Geometry: final body of the model. Coordinates: model frame, mm. A direction names the side the tool comes from. Round coordinates to 2 decimals unless told otherwise and drop trailing zeros. Order: outer loops, then holes, each group sorted by start corner. A loop starts at its lowest first (then second) coordinate and runs counter-clockwise, first axis right, second up. Notation, with made-up numbers: M -37.5,-28.5 L -24.5,-28.5 A21 ccw -24.5,-11.5 Z; hole C 85.25,-30 d2. An arc over 180 degrees is marked long. Put each result on its own line as item: value. Start each with the question number.
1) Section C-C, the plane y = 13. Return loops of the section in (x, z).
2) Section B-B, the plane z = -8.75. Return loops of the section in (x, y).
3) First-contact query: P1, Ø6, axis at y = 26, z = -4, coming from the -X side; P2, Ø1.2, axis at x = 1.5, y = 32.5, coming from the -Z side; P3, Ø4, axis at y = 7.5, z = -12.2, coming from the -X side. Flat tips, straight axial feed; report the tip coordinate or a pass-through.
4) Material intervals for probe 1 along Y at (x, z) = (1.2, -7.5); probe 2 along Z at (x, y) = (-1.1, 20); probe 3 along Y at (x, z) = (1.4, -13), sorted ascending. Write a range as [from, to].
5) Section D-D, the plane x = -0.45. Return loops of the section in (y, z), then the cut area to 3 significant figures.
6) Access query for faces 4 (the flat face through (1.232, 34.936, -13.58)), 5 (the flat face through (1, 7, -9.4)), 6 (the cylindrical face through (-3.01, 4.96, -12.76)). Directions: +Z, -Z, +X, -X, +Y, -Y. A direction counts if a zero-diameter tool reaches every point of the face in a straight line with its end or side. Return the directions, or none.
7) Draft query along Z for faces 1 (the flat face through (1.232, 34.914, -10.78)), 2 (the flat face through (-2.5, 20.3, -5.7)), 3 (the flat face through (1, 32, -9.4)). Return one class per face: pulls with the +Z half, pulls with the -Z half, needs draft (parallel to the pull), parting line crosses it, or undercut.
8) Section A-A, the plane x = 1.2. Return loops of the section in (y, z), then the cut area to 3 significant figures.
from build123d import *
from build123d.topology import SkipClean

# Parameters (mm, degrees)
BOSS_EXTRUDE1_DEPTH = 2.5
BOSS_EXTRUDE2_START = -2.5
SKETCH1_3_W         = 15
SKETCH1_3_H         = 40
SKETCH1_3_R         = 1.6
BOSS_EXTRUDE2_DEPTH = 2.5
EXTRUDE_THIN1_START = 1
SKETCH2_R           = 2.6
SKETCH2_R_2         = 1.6
EXTRUDE_THIN1_DEPTH = 1
CUT_EXTRUDE1_DEPTH  = 2.5


with BuildPart() as part:
    # Sketch1 → Boss-Extrude1 (new body)
    with BuildSketch(Plane(origin=(0, 0, 0), x_dir=(0, 0, -1), z_dir=(1, 0, 0))):
        with BuildLine():
            Line((7.5, 21.6), (7.5, 40))
            Line((7.5, 40), (0, 40))
            Line((0, 40), (0, 0))
            Line((0, 0), (7.5, 0))
            Line((7.5, 0), (7.5, 6.4))
            ThreePointArc((7.5, 6.4), (5.9, 8), (7.5, 9.6))
            Line((7.5, 9.6), (7.5, 18.4))
            ThreePointArc((7.5, 18.4), (5.9, 20), (7.5, 21.6))
        make_face()
        with BuildLine():
            Line((15, 40), (7.5, 40))
            Line((7.5, 40), (7.5, 21.6))
            ThreePointArc((7.5, 21.6), (8.63137085, 21.13137085), (9.1, 20))
            ThreePointArc((9.1, 20), (8.63137085, 18.86862915), (7.5, 18.4))
            Line((7.5, 18.4), (7.5, 9.6))
            ThreePointArc((7.5, 9.6), (8.63137085, 9.13137085), (9.1, 8))
            ThreePointArc((9.1, 8), (8.63137085, 6.86862915), (7.5, 6.4))
            Line((7.5, 6.4), (7.5, 0))
            Line((7.5, 0), (15, 0))
            Line((15, 0), (15, 5.883419246))
            Line((15, 5.883419246), (12.2, 4.266838493))
            Line((12.2, 4.266838493), (9.4, 5.883419246))
            Line((9.4, 5.883419246), (9.4, 9.116580754))
            Line((9.4, 9.116580754), (12.2, 10.733161507))
            Line((12.2, 10.733161507), (15, 9.116580754))
            Line((15, 9.116580754), (15, 30.883419246))
            Line((15, 30.883419246), (12.2, 29.266838493))
            Line((12.2, 29.266838493), (9.4, 30.883419246))
            Line((9.4, 30.883419246), (9.4, 34.116580754))
            Line((9.4, 34.116580754), (12.2, 35.733161507))
            Line((12.2, 35.733161507), (15, 34.116580754))
            Line((15, 34.116580754), (15, 40))
        make_face()
        with BuildLine():
            ThreePointArc((9.1, 8), (8.63137085, 9.13137085), (7.5, 9.6))
            Line((7.5, 9.6), (7.5, 6.4))
            ThreePointArc((7.5, 6.4), (8.63137085, 6.86862915), (9.1, 8))
        make_face()
        with BuildLine():
            Line((7.5, 6.4), (7.5, 9.6))
            ThreePointArc((7.5, 9.6), (5.9, 8), (7.5, 6.4))
        make_face()
    extrude(amount=BOSS_EXTRUDE1_DEPTH)

    # Sketch1_3 → Boss-Extrude2 (add)
    with SkipClean():  # the faces are left unmerged after this step: merging them gives an invalid solid
        with BuildSketch(Plane(origin=(0, 0, 0), x_dir=(0, 0, -1), z_dir=(1, 0, 0)).offset(BOSS_EXTRUDE2_START)):
            with Locations((7.5, 20)):
                Rectangle(SKETCH1_3_W, SKETCH1_3_H)
            with Locations((7.5, 20)):
                Circle(SKETCH1_3_R, mode=Mode.SUBTRACT)
            with Locations((12.2, 32.5)):
                Circle(SKETCH1_3_R, mode=Mode.SUBTRACT)
            with Locations((12.2, 7.5)):
                Circle(SKETCH1_3_R, mode=Mode.SUBTRACT)
        extrude(amount=BOSS_EXTRUDE2_DEPTH)

    # Sketch2 → Extrude-Thin1 (add)
    # profile 1 of 2: a face of its own
    with SkipClean():  # the faces are left unmerged after this step: merging them gives an invalid solid
        with BuildSketch(Plane.ZY.offset(2.5).offset(EXTRUDE_THIN1_START)):
            with Locations((-12.2, 7.5)):
                Circle(SKETCH2_R)
            with Locations((-12.2, 7.5)):
                Circle(SKETCH2_R_2, mode=Mode.SUBTRACT)
        # profile 2 of 2: a face of its own
        with BuildSketch(Plane.ZY.offset(2.5).offset(EXTRUDE_THIN1_START)):
            with Locations((-12.2, 32.5)):
                Circle(SKETCH2_R)
            with Locations((-12.2, 32.5)):
                Circle(SKETCH2_R_2, mode=Mode.SUBTRACT)
        extrude(amount=-EXTRUDE_THIN1_DEPTH)

    # Sketch3 → Cut-Extrude1 (cut)
    with SkipClean():  # the faces are left unmerged after this step: merging them gives an invalid solid
        with BuildSketch(Plane.ZY.offset(2.5)):
            with BuildLine():
                ThreePointArc((0, 33.564659966), (-2.979157617, 27.071067812), (-4, 20))
                Line((-4, 20), (0, 20))
                Line((0, 20), (0, 33.564659966))
            make_face()
            with BuildLine():
                Line((0, 20), (-4, 20))
                ThreePointArc((-4, 20), (-2.979157617, 12.928932188), (0, 6.435340034))
                Line((0, 6.435340034), (0, 20))
            make_face()
            with BuildLine():
                Line((0, 33.564659966), (0, 20))
                Line((0, 20), (0, 6.435340034))
                ThreePointArc((0, 6.435340034), (28.071067812, -3.979157617), (46, 20))
                ThreePointArc((46, 20), (28.071067812, 43.979157617), (0, 33.564659966))
            make_face()
        extrude(amount=-CUT_EXTRUDE1_DEPTH, mode=Mode.SUBTRACT)


solid = part.part
Result sheet:
1. outline: M -2.5,-15 L 2.5,-15 L 2.5,0 L 0,0 L 0,-3 L -2.5,-3 Z
2. outline: M -2.5,0 L 2.5,0 L 2.5,19 L -2.5,19 Z; M -2.5,21 L 2.5,21 L 2.5,40 L -2.5,40 Z
3. P1: stops at x = -2.5
3. P2: stops at z = -9.4
3. P3: stops at x = -3.5
4. probe 1: y = [0, 18.4], [21.6, 40]
4. probe 2: z = [-15, -9.1], [-5.9, -4]
4. probe 3: y = [0, 4.73], [10.27, 29.73], [35.27, 40]
5. outline: M 0,-15 L 40,-15 L 40,0 L 33.56,0 A25 cw 6.44,0 L 0,0 Z; hole C 7.5,-12.2 d3.2; hole C 20,-7.5 d3.2; hole C 32.5,-12.2 d3.2
5. area: 502 mm2
6. face 4: +X
6. face 5: -Z, +X
6. face 6: -X
7. face 1: undercut
7. face 2: needs draft
7. face 3: pulls with the -Z half
8. outline: M 0,-15 L 5.88,-15 L 4.27,-12.2 L 5.88,-9.4 L 9.12,-9.4 L 10.73,-12.2 L 9.12,-15 L 30.88,-15 L 29.27,-12.2 L 30.88,-9.4 L 34.12,-9.4 L 35.73,-12.2 L 34.12,-15 L 40,-15 L 40,0 L 0,0 Z; hole C 20,-7.5 d3.2
8. area: 538 mm2
